The listing builds one solid part. Answer for the finished solid, in the listing's coordinates (mm). Face numbers are marked on the shaded views. A direction names the side the tool comes from. Round coordinates to 2 decimals unless told otherwise and drop trailing zeros. Loops run counter-clockwise (first coordinate to the right, second up) from the corner with the lowest first, then second, coordinate; pieces in that order, holes last. Notation, with made-up numbers: (74.25, 3) -> (99.25, 3) arc R13 ccw to (99.25, 13) -> close; hole circle Ø10 at (40, -9.5). An arc over 180 degrees is marked (long way). Write each question's results on one line, items separated by ' | '. Start each with the question number.
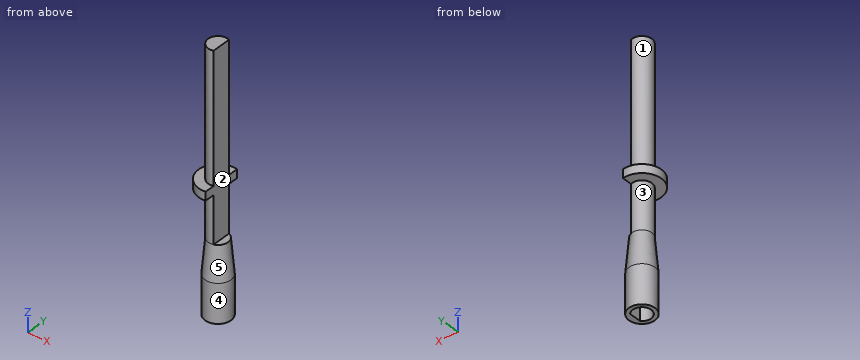
from build123d import *

# Parameters (mm, degrees)
BOSS_EXTRUDE2_DEPTH      = 2
BOSS_EXTRUDE3_DEPTH      = 30
BOSS_EXTRUDE3_DEPTH_BACK = 30
SKETCH3_R                = 3
BOSS_EXTRUDE4_DEPTH      = 17
CUT_EXTRUDE1_DEPTH       = 7.5


with BuildPart() as part:
    # Sketch2 → Boss-Extrude2 (new body)
    with BuildSketch(Plane.XY):
        with BuildLine():
            Line((0.762299154, -4.434963359), (0.762299154, 4.434963359))
            ThreePointArc((0.762299154, 4.434963359), (-4.5, 0), (0.762299154, -4.434963359))
        make_face()
    extrude(amount=-BOSS_EXTRUDE2_DEPTH)

    # Sketch1 → Boss-Extrude3 (add, two sides)
    with BuildSketch(Plane.XY) as boss_extrude3_sk:
        with BuildLine():
            Line((0.762299154, -2.17), (0.762299154, 2.17))
            ThreePointArc((0.762299154, 2.17), (-2.3, 0), (0.762299154, -2.17))
        make_face()
    extrude(amount=BOSS_EXTRUDE3_DEPTH)
    extrude(boss_extrude3_sk.sketch, amount=-BOSS_EXTRUDE3_DEPTH_BACK)

    # Sketch3 → Boss-Extrude4 (add)
    with BuildSketch(Plane(origin=(0, 0, -30), x_dir=(-1, 0, 0), z_dir=(0, 0, -1))):
        Circle(SKETCH3_R)
    extrude(amount=-BOSS_EXTRUDE4_DEPTH)

    # Sketch4 → Cut-Extrude1 (cut)
    with BuildSketch(Plane(origin=(0, 0, -30), x_dir=(-1, 0, 0), z_dir=(0, 0, -1))):
        with BuildLine():
            Line((-1.59, 1.409796085), (-1.59, -1.409796085))
            ThreePointArc((-1.59, -1.409796085), (2.125, 0), (-1.59, 1.409796085))
        make_face()
    extrude(amount=-CUT_EXTRUDE1_DEPTH, mode=Mode.SUBTRACT)

    # Sketch7 → Cut-Revolve1 (revolve, cut)
    with BuildSketch(Plane(origin=(0, 0, 0), x_dir=(0, 0, -1), z_dir=(1, 0, 0))):
        Polygon((13, 3), (21, 3), (13, 2.3), align=None)
    revolve(axis=Axis((0, 0, 30.362206594), (0, 0, -1)), mode=Mode.SUBTRACT)


solid = part.part
Item 1: The part is cut by section C-C, the plane z = 10.5. Give the vertices of the cut face in (x, y).
Item 2: Each of these flat-tipped pins is pushed along its axis until it touches: pin 1 Ø2 at (y, z) = (-3, -5) entering from -X; pin 2 Ø1.4 at (y, z) = (-0.5, -27) entering from -X; pin 3 Ø2 at (x, y) = (-3.5, -2) entering from +Z. Where does it stop, or does it pass through?
Item 3: The part is cut by section B-B, the plane y = 0. Give the vertices of the cut face in (x, z) (3 decimals), plus the area to 3 significant figures.
Item 4: Determine the mould class of the marked faces 4 and 5 for opening direction Z: +Z half, -Z half, draft (parallel to the pull), parting line (faces both ways), or undercut.
Item 5: Straight lines are drawn through the part: L1, parallel to Z at x = -1.75, y = -0.5; L2, parallel to Z at x = -1.75, y = -3; L3, parallel to X at y = -0.75, z = 23.5. For each, find the intervals that lie inside material, in ascending order. Write a range as [from, to].
Item 6: The part is cut by section A-A, the plane x = 0. Give the vertices of the cut face in (y, z) (3 decimals), plus the area to 3 significant figures.
Item 7: For the marked faces 1, 2 and 3, determine the directions among +Z, -Z, +X, -X, +Y, -Y from which every point of the face is accessible in a straight line to the end or side of a thin tool.
Item 8: The part is cut by section D-D, the plane z = -20.5. Give the vertices of the cut face in (x, y), plus the area to 3 significant figures.
Report:
1) outline: (0.76, -2.17) -> (0.76, 2.17) arc R2.3 ccw (long way) to start
2) pin 1: stops at x = -1.14 | pin 2: stops at x = -3 | pin 3: stops at z = 0
3) outline: (-4.5, -2) -> (-2.3, -2) -> (-2.3, -13) -> (-3, -21) -> (-3, -30) -> (-2.125, -30) -> (-2.125, -22.5) -> (1.59, -22.5) -> (1.59, -30) -> (3, -30) -> (3, -21) -> (2.3, -13) -> (0.762, -13) -> (0.762, 30) -> (-2.3, 30) -> (-2.3, 0) -> (-4.5, 0) -> close | area: 205 mm2
4) face 4: draft | face 5: undercut
5) L1: z = [-22.5, 30] | L2: z = [-2, 0] | L3: x = [-2.17, 0.76]
6) outline: (-4.5, -2) -> (-2.3, -2) -> (-2.3, -13) -> (-3, -21) -> (-3, -30) -> (-2.125, -30) -> (-2.125, -22.5) -> (2.125, -22.5) -> (2.125, -30) -> (3, -30) -> (3, -21) -> (2.3, -13) -> (2.3, -2) -> (4.5, -2) -> (4.5, 0) -> (2.3, 0) -> (2.3, 30) -> (-2.3, 30) -> (-2.3, 0) -> (-4.5, 0) -> close | area: 271 mm2
7) face 1: +Z | face 2: +Z, +X, +Y, -Y | face 3: none
8) outline: circle Ø5.91 at (0, 0) | area: 27.5 mm2
